CAD build for the part. Positions are in the model's coordinates, mm. A direction names the side the tool comes from. Round coordinates to 2 decimals unless told otherwise and drop trailing zeros. Order: outer loops, then holes, each group sorted by start corner. A loop starts at its lowest first (then second) coordinate and runs counter-clockwise, first axis right, second up. Notation, with made-up numbers: M 1.25,10 L 5.25,10 A14 ccw 5.25,16 Z; hole C 26.5,-33.75 d6. An arc over 180 degrees is marked long. Answer as a JSON object with one key per item and string values. Group by question number.
```python
from build123d import *
from build123d import SkipClean  # not in build123d's __all__

# Parameters (mm, degrees)
F0_R     = 5
F1_DEPTH = 33
F2_W     = 9
F2_H     = 19
F3_DEPTH = 140
F5_DEPTH = 33


with BuildPart() as f1:
    # F0 (on Right) → F1 (new body)
    with BuildSketch(Plane.YZ):
        with BuildLine():
            ThreePointArc((0, 8), (35.2278299076, 5.9935116916), (70, 0))
            Line((70, 0), (70, 7.1810302798))
            ThreePointArc((70, 7.1810302798), (37.1952808389, 12.8120154562), (3.9811421818, 14.975019516))
            ThreePointArc((3.9811421818, 14.975019516), (2.2220595829, 13.5208872296), (0, 13))
            Line((0, 13), (0, 8))
        make_face()
        with BuildLine():
            ThreePointArc((3.9811421818, 14.975019516), (37.1952808389, 12.8120154562), (70, 7.1810302798))
            Line((70, 7.1810302798), (70, 26))
            Line((70, 26), (0, 26))
            Line((0, 26), (0, 23))
            ThreePointArc((0, 23), (3.5355339059, 21.5355339059), (5, 18))
            ThreePointArc((5, 18), (4.7384444129, 16.4040223856), (3.9811421818, 14.975019516))
        make_face()
        with Locations((55, 18)):
            Circle(F0_R, mode=Mode.SUBTRACT)
        with BuildLine():
            Line((-70, 26), (-70, 7.1810302798))
            ThreePointArc((-70, 7.1810302798), (-37.1952808389, 12.8120154562), (-3.9811421818, 14.975019516))
            ThreePointArc((-3.9811421818, 14.975019516), (-4.4791127704, 20.2220595829), (0, 23))
            Line((0, 23), (0, 26))
            Line((0, 26), (-70, 26))
        make_face()
        with Locations((-55, 18)):
            Circle(F0_R, mode=Mode.SUBTRACT)
        with BuildLine():
            Line((-70, 7.1810302798), (-70, 0))
            ThreePointArc((-70, 0), (-35.2278299076, 5.9935116916), (0, 8))
            Line((0, 8), (0, 13))
            ThreePointArc((0, 13), (-2.2220595829, 13.5208872296), (-3.9811421818, 14.975019516))
            ThreePointArc((-3.9811421818, 14.975019516), (-37.1952808389, 12.8120154562), (-70, 7.1810302798))
        make_face()
    extrude(amount=F1_DEPTH)

    # F2 (on face) → F3 (cut)
    with BuildSketch(Plane.XZ.offset(70)):
        with Locations((16.5, 16.5)):
            Rectangle(F2_W, F2_H)
    extrude(amount=-F3_DEPTH, mode=Mode.SUBTRACT)

    # F4 (on face) → F5 (join)
    with BuildSketch(Plane.YZ.offset(33)):
        with BuildLine():
            Line((70, 0), (70, 7.1810302798))
            ThreePointArc((70, 7.1810302798), (37.1952808389, 12.8120154562), (3.9811421818, 14.975019516))
            ThreePointArc((3.9811421818, 14.975019516), (0, 13), (-3.9811421818, 14.975019516))
            ThreePointArc((-3.9811421818, 14.975019516), (-37.1952808389, 12.8120154562), (-70, 7.1810302798))
            Line((-70, 7.1810302798), (-70, 0))
            ThreePointArc((-70, 0), (0, 8), (70, 0))
        make_face()
    with SkipClean():  # cleaning this boolean's faces spoils the solid; the shape is the same uncleaned
        extrude(amount=-F5_DEPTH)


solid = f1.part
```
Item 1: Cut at C-C, the plane x = 28. Give the cut face in (y, z), and give its area (3 significant figures).
Item 2: Two-plate mould, pull along Z, no slides. Class faces 4 (the face through (6, -59, 15)), 5 (the face through (27, -59, 15)), 6 (the face through (16, -1, 8)), 7 (the face through (24, -70, 13)): +Z half, -Z half, draft (parallel to the pull), parting line (faces both ways), or undercut.
Item 3: Drill centre lines: line 1 (Y direction, x = 30, z = 18); line 2 (X direction, y = 22, z = 23.25); line 3 (Z direction, x = 29.75, y = 55). Where is each one in solid material? Low to high. Write a range as [from, to].
Item 4: Cut at D-D, the plane y = -43. Give the cut face in (x, z), and give its area (3 significant figures).
Item 5: Cut at A-A, the plane z = 18. Give the number of separate pieces and of enclosed holes in the cut face, and give its area (3 significant figures).
Item 6: 3-axis set-ups, long thin cutter, end or side, ignore diameter. For faces 1 (the face through (16.563, -36.732, 12.866)), 2 (the face through (16.563, 37.658, 12.757)), 3 (the face through (5.92, 53.92, 13.12)): which of +Z, -Z, +X, -X, +Y, -Y reach the whole face in a straight line?
Item 7: Flat gauge pin, fed straight in: pin 1 Ø8 at (y, z) = (-55, 18) entering from -X. Where does the tip first touch, or does it go through?
Item 8: Cut at B-B, the plane y = 0. Give the cut face in (x, z).
Response values:
{
 "1": {"outline": "M -70,0 A310.25 cw 70,0 L 70,26 L -70,26 Z; hole C -55,18 d10; hole C 0,18 d10; hole C 55,18 d10", "area": "2,660 mm^2"},
 "2": {"face 4": "undercut", "face 5": "undercut", "face 6": "-Z half", "face 7": "draft"},
 "3": {"line 1": "[-70, -60], [-50, -5], [5, 50], [60, 70]", "line 2": "[0, 12], [21, 33]", "line 3": "[3.09, 13], [23, 26]"},
 "4": {"outline": "M 0,5.01 L 33,5.01 L 33,26 L 21,26 L 21,12.07 L 12,12.07 L 12,26 L 0,26 Z", "area": "567 mm^2"},
 "5": {"separate pieces": "8", "enclosed holes": "0", "area": "2,640 mm^2"},
 "6": {"face 1": "+Z, -Y", "face 2": "+Z, +Y", "face 3": "+X, -X"},
 "7": {"pin 1": "through"},
 "8": {"outline": "M 0,8 L 33,8 L 33,13 L 0,13 Z; M 0,23 L 12,23 L 12,26 L 0,26 Z; M 21,23 L 33,23 L 33,26 L 21,26 Z"}
}
